Verification items for the finished model (mm, model axes). Face numbers are marked on the shaded views. A direction names the side the tool comes from. Give positions to 0.01 mm unless a question says otherwise; leave off trailing zeros. Loops run counter-clockwise (first coordinate to the right, second up) from the corner with the lowest first, then second, coordinate; pieces in that order, holes last. Notation, with made-up numbers: (34.5, 37) -> (54.5, 37) arc R12 ccw to (54.5, 46) -> close; hole circle Ø7 at (20, 30.25). An arc over 180 degrees is marked (long way). Answer in a Markdown table with one row per item. Add a question column.
Q1. Section check A-A on y = 0. Enter the section's corners in (x, z), and give its area (3 significant figures).
Q2. Gauge pin test, flat ends, axial feed: P1, Ø1.7, axis at x = 6, y = 0, coming from the -Z side; P2, Ø2.5, axis at x = 0.5, z = 2.5, coming from the -Y side; P3, Ø2.5, axis at x = -0.5, z = 5.5, coming from the +Y side; P4, Ø3, axis at x = -3, z = 8, coming from the -Y side. Record the tip position at first contact, or that the pin passes through.
Q3. Material ranges on probe 1 along X at (y, z) = (-1.25, 5.5); probe 2 along X at (y, z) = (-0.5, 1.5); probe 3 along Y at (x, z) = (6, 5.75), recorded low to high.
Q4. Section check C-C on z = 4. Enter the section's corners in (x, y).
Q5. Set-up check for the marked faces 5 and 6: record each of +Z, -Z, +X, -X, +Y, -Y from which the full face is reachable in a straight line by a thin tool's end or side.
Q6. Section check B-B on x = -6. Enter the section's corners in (y, z).
Q7. Section check D-D on y = 3. Enter the section's corners in (x, z), and give its area (3 significant figures).
Q8. Release check for a two-part mould opening along Y. For the marked faces 1, 2, 3 and 4 record: pulls with the +Y half, pulls with the -Y half, needs draft (parallel to the pull), parting line crosses it, or undercut.
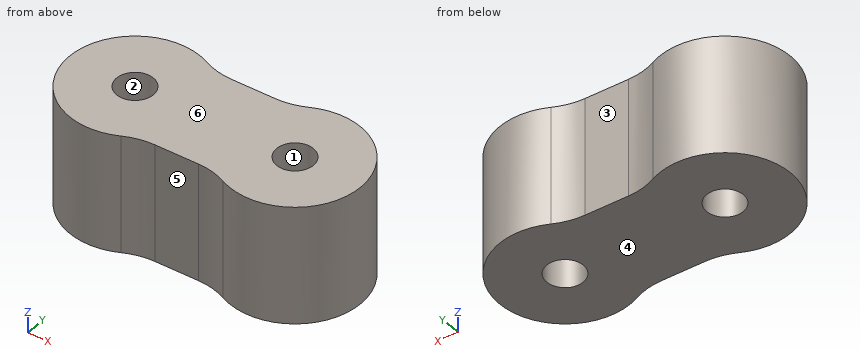
```python
from build123d import *

# Parameters (mm, degrees)
F0_R     = 1.4
F1_DEPTH = 9
F2_R     = 5


with BuildPart() as f1:
    # F0 (on Top) → F1 (new body)
    with BuildSketch(Plane.XY):
        with BuildLine():
            Line((0, -4), (0, 0))
            Line((0, 0), (-1, 0))
            ThreePointArc((-1, 0), (-1.527864, -2.236068), (-3, -4))
            Line((-3, -4), (0, -4))
        make_face()
        with BuildLine():
            Line((-1, 0), (0, 0))
            Line((0, 0), (0, 4))
            Line((0, 4), (-3, 4))
            ThreePointArc((-3, 4), (-1.527864, 2.236068), (-1, 0))
        make_face()
        with Locations((-6, 0)):
            Circle(F0_R)
        with BuildLine():
            ThreePointArc((-3, -4), (-1.527864, -2.236068), (-1, 0))
            ThreePointArc((-1, 0), (-1.527864, 2.236068), (-3, 4))
            ThreePointArc((-3, 4), (-11, 0), (-3, -4))
        make_face()
        with Locations((-6, 0)):
            Circle(F0_R, mode=Mode.SUBTRACT)
    extrude(amount=F1_DEPTH)

    # F2
    f2_edges = [f1.edges().sort_by_distance(p)[0] for p in [
        (-3, 4, 4.5),
        (-3, -4, 4.5),
    ]]
    fillet(f2_edges, radius=F2_R)

    # F3: F1 across face


with BuildPart() as f1_1:
    add(f1.part)
    add(f1.part.mirror(Plane(origin=(0, 0, 4.5), x_dir=(0, 1, 0), z_dir=(1, 0, 0))))


solid = f1_1.part
```
Taken from the geometry:
| question | item | result |
|---|---|---|
| 1 | outline | (-11, 0) -> (-7.4, 0) -> (-7.4, 9) -> (-11, 9) -> close; (-4.6, 0) -> (4.6, 0) -> (4.6, 9) -> (-4.6, 9) -> close; (7.4, 0) -> (11, 0) -> (11, 9) -> (7.4, 9) -> close |
| 1 | area | 148 mm² |
| 2 | P1 | passes through |
| 2 | P2 | stops at y = -4 |
| 2 | P3 | stops at y = 4 |
| 2 | P4 | stops at y = -4.77 |
| 3 | probe 1 | x = -10.84 to -6.63, -5.37 to 5.37, 6.63 to 10.84 |
| 3 | probe 2 | x = -10.97 to -7.31, -4.69 to 4.69, 7.31 to 10.97 |
| 3 | probe 3 | y = -5 to -1.4, 1.4 to 5 |
| 4 | outline | (-3.82, -4.5) arc R5 cw to (-1.64, -4) -> (1.64, -4) arc R5 cw to (3.82, -4.5) arc R5 ccw (long way) to (3.82, 4.5) arc R5 cw to (1.64, 4) -> (-1.64, 4) arc R5 cw to (-3.82, 4.5) arc R5 ccw (long way) to start; hole circle Ø2.8 at (-6, 0); hole circle Ø2.8 at (6, 0) |
| 5 | face 5 | +Z, -Z, -Y |
| 5 | face 6 | +Z, +X, -X, +Y, -Y |
| 6 | outline | (-5, 0) -> (-1.4, 0) -> (-1.4, 9) -> (-5, 9) -> close; (1.4, 0) -> (5, 0) -> (5, 9) -> (1.4, 9) -> close |
| 7 | outline | (-10, 0) -> (10, 0) -> (10, 9) -> (-10, 9) -> close |
| 7 | area | 180 mm² |
| 8 | face 1 | undercut |
| 8 | face 2 | undercut |
| 8 | face 3 | pulls with the +Y half |
| 8 | face 4 | needs draft |
